Here's how the part is built. I have some questions about the finished solid (model axes, mm). Give positions to 0.01 mm unless a question says otherwise; leave off trailing zeros. Write each loop counter-clockwise with the first axis right and the second up, starting at its lowest first coordinate (ties: lowest second). Pieces come first, ordered by that corner, then holes. Notation, with made-up numbers: (76, 15) -> (92, 15) arc R23 cw to (92, 43) -> close; hole circle Ø8 at (68.5, -35). An arc over 180 degrees is marked (long way). Put each result on its own line as item: value. Start each with the question number.
from build123d import *

# Parameters (mm, degrees)
SKETCH1_R                   = 63.5
BOSS_EXTRUDE1_DEPTH         = 3.175
TAP_DRILL_FOR_M4X0_7_TAP1_D = 3.3
F_9_0_196_DIAMETER_HOLE1_D  = 4.9784
CUT_EXTRUDE1_DEPTH          = 90.858670283
CUT_EXTRUDE1_DEPTH_BACK     = 90.858670283
SKETCH12_R                  = 3.2639
SKETCH12_R_2                = 1.65


with BuildPart() as part:
    # Sketch1 → Boss-Extrude1 (new body)
    with BuildSketch(Plane(origin=(0, 0, 0), x_dir=(1, 0, 0), z_dir=(0, 1, 0))):
        with Locations(Location((0, 0, 0), (0, 0, 270))):
            Circle(SKETCH1_R)
    extrude(amount=BOSS_EXTRUDE1_DEPTH)

    # Tap Drill for M4x0.7 Tap1 (through all)
    with Locations(Plane(origin=(0, 3.175, 0), x_dir=(1, 0, 0), z_dir=(0, 1, 0))):
        with Locations((0, 34), (0, -34)):
            Hole(TAP_DRILL_FOR_M4X0_7_TAP1_D / 2)

    # #9 (0.196) Diameter Hole1 (through all)
    with Locations(Plane(origin=(0, 3.175, 0), x_dir=(1, 0, 0), z_dir=(0, 1, 0))):
        with Locations((14.791508428, 55.202660972), (57.15, 0), (14.791508428, -55.202660972)):
            Hole(F_9_0_196_DIAMETER_HOLE1_D / 2)

    # Sketch12 → Cut-Extrude1 (cut, two sides: drawn at the far end of the back side and taken through both)
    with BuildSketch(Plane(origin=(0, 3.175, 0), x_dir=(1, 0, 0), z_dir=(0, 1, 0)).offset(-CUT_EXTRUDE1_DEPTH_BACK)):
        with Locations(Location((-34.925, 0, 0), (0, 0, 270))):
            Circle(SKETCH12_R)
        with Locations(Location((-34.925, 17.9999894, 0), (0, 0, 270))):
            Circle(SKETCH12_R_2)
        with Locations(Location((-34.925, -17.9999894, 0), (0, 0, 270))):
            Circle(SKETCH12_R_2)
        with Locations(Location((19.05, 34, 0), (0, 0, 270))):
            Circle(SKETCH12_R_2)
        with Locations(Location((19.05, -34, 0), (0, 0, 270))):
            Circle(SKETCH12_R_2)
    extrude(amount=CUT_EXTRUDE1_DEPTH + CUT_EXTRUDE1_DEPTH_BACK, mode=Mode.SUBTRACT)


solid = part.part
1) I want a section at A-A, the plane x = 0. Write out the boundary of the cut face in (y, z) (3 decimals).
2) I want a section at C-C, the plane y = 1.4. State how many separate pieces and enclosed holes the cut face has, and give its area (3 significant figures).
3) I need wall thicknesses on probe 1 along X at (y, z) = (1.5, -34); probe 2 along Z at (x, y) = (19.05, 1.85); probe 3 along X at (y, z) = (1.9, -0.5). Which ranges of each line are inside material? Lowest first, please.
4) Thinking about a two-plate mould opening in X: for faces 1 (the flat face through (1, 3.175, -1)), 2 (the cylindrical face through (-0.89, 1.57, -35.39)), 3 (the cylindrical face through (-61.99, 1.57, -13.77)), which applies, released by +X, released by -X, zero draft, split by the parting line, or undercut?
5) I'm going to push a flat-ended pin straight in: pin 1 Ø3 at (x, z) = (19.05, 34) entering from -Y. Where does the tip first touch, or does it pass through?
6) I want a section at D-D, the plane x = 57.15. Write out the boundary of the cut face in (y, z) (3 decimals), and give its area (3 significant figures).
7) I want a section at B-B, the plane z = 0. Write out the boundary of the cut face in (x, y) (3 decimals), and give its area (3 significant figures).
Established:
1. outline: (0, -63.5) -> (3.175, -63.5) -> (3.175, -35.65) -> (0, -35.65) -> close; (0, -32.35) -> (3.175, -32.35) -> (3.175, 32.35) -> (0, 32.35) -> close; (0, 35.65) -> (3.175, 35.65) -> (3.175, 63.5) -> (0, 63.5) -> close
2. separate pieces: 1
2. enclosed holes: 10
2. area: 12,500 mm2
3. probe 1: x = -53.63 to -1.65, 1.65 to 17.4, 20.7 to 53.63
3. probe 2: z = -60.58 to -35.65, -32.35 to 32.35, 35.65 to 60.58
3. probe 3: x = -63.5 to -38.15, -31.7 to 54.71, 59.59 to 63.5
4. face 1: zero draft
4. face 2: undercut
4. face 3: split by the parting line
5. pin 1: passes through
6. outline: (0, -27.679) -> (3.175, -27.679) -> (3.175, -2.489) -> (0, -2.489) -> close; (0, 2.489) -> (3.175, 2.489) -> (3.175, 27.679) -> (0, 27.679) -> close
6. area: 160 mm2
7. outline: (-63.5, 0) -> (-38.189, 0) -> (-38.189, 3.175) -> (-63.5, 3.175) -> close; (-31.661, 0) -> (54.661, 0) -> (54.661, 3.175) -> (-31.661, 3.175) -> close; (59.639, 0) -> (63.5, 0) -> (63.5, 3.175) -> (59.639, 3.175) -> close
7. area: 367 mm2
